```python
from build123d import *

# Parameters (mm, degrees)
F1_DEPTH    = 130
F2_T1_DEPTH = 154.4948974279
F3_T1_DEPTH = 154.4948974279
F4_R        = 5


# Not quite as in the source:
# - a fillet or chamfer that OpenCascade refuses, or shapes differently, is made with other operations: its cross-section is extruded or revolved along the edge and cut away or added


with BuildPart() as f1:
    # F0 (on Right) → F1 (new body)
    with BuildSketch(Plane.YZ):
        Polygon((1.0352761804, 3.8637033052), (0, 0), (120, 0), (120, 4), (5.2129014914, 4), (30.6586225483, 98.9647238196), (26.7949192431, 100), align=None)
        Polygon((-10, 0), (0, 0), (1.0352761804, 3.8637033052), (-10, 6.820596646), (-10, 4.0079755444), align=None)
    extrude(amount=F1_DEPTH)

    # F2: fillet of radius 5 on 1 edges, made by hand

    # F2_s2 → F2_t1 (cut)
    with BuildSketch(Plane.YZ.offset(-12.2474487139)):
        with BuildLine():
            ThreePointArc((30.6586225483, 98.9647238196), (27.4340422276, 98.0307814801), (25.5269700507, 95.2679491924))
            Line((25.5269700507, 95.2679491924), (26.7949192431, 100))
            Line((26.7949192431, 100), (30.6586225483, 98.9647238196))
        make_face()
    extrude(amount=F2_T1_DEPTH, mode=Mode.SUBTRACT)

    # F3: fillet of radius 5 on 1 edges, made by hand

    # F3_s2 → F3_t1 (cut)
    with BuildSketch(Plane.YZ.offset(-12.2474487139)):
        with BuildLine():
            ThreePointArc((115.1010205144, 4), (118.2632981746, 2.8729833462), (120, 0))
            Line((120, 0), (120, 4))
            Line((120, 4), (115.1010205144, 4))
        make_face()
    extrude(amount=F3_T1_DEPTH, mode=Mode.SUBTRACT)

    # F4
    f4_edges = [f1.edges().sort_by_distance(p)[0] for p in [
        (65, -10, 6.820597),
    ]]
    fillet(f4_edges, radius=F4_R)


solid = f1.part
```
Model file for the job. Use its own axes, mm. A direction names the side the tool comes from. Give positions to 0.01 mm unless a question says otherwise; leave off trailing zeros. Loops run counter-clockwise (first coordinate to the right, second up) from the corner with the lowest first, then second, coordinate; pieces in that order, holes last. Notation, with made-up numbers: (14, 14) -> (36, 14) arc R14 ccw to (36, 32) -> close; hole circle Ø1 at (-28.5, -13.5). An arc over 180 degrees is marked (long way). Use CSV: the item, a comma, the result in double quotes. Start each with the question number.
1) Slice it at A-A on x = 74. Give the cut face in (y, z).
2) Slice it at D-D on z = 22. Give the cut face in (x, y).
3) Tool access for faces 4 (the flat face through (0, 35, 2)), 5 (the flat face through (64.09, -1.3, 4.49)), 6 (the flat face through (64.09, 17.76, 50.82)): list every direction of +Z, -Z, +X, -X, +Y, -Y with a clear straight run to the whole face (end or side of a thin tool).
4) Flat gauge pins, fed straight in: pin 1 Ø3 at (x, y) = (36, 96.5) entering from +Z; pin 2 Ø4 at (x, z) = (97.5, 20.5) entering from +Y; pin 3 Ø3 at (x, z) = (70, 53) entering from -Y. Where does each tip first touch, or does it go through?
5) Mould opens along Z. For faces 1 (the flat face through (64, 61, 4)), 2 (the flat face through (64, 54, 0)), 3 (the cylindrical face through (64.09, 118.23, 2.9)) say: released by +Z, released by -Z, zero draft, split by the parting line, or undercut.
6) Slice it at B-B on y = 7. Give the cut face in (x, z), plus the area to 3 significant figures.
7) Slice it at C-C on y = 56. Give the cut face in (x, z).
8) Wall check: line 1 (Z direction, x = 86.5, y = 86); line 2 (Y direction, x = 78, z = 47); line 3 (Y direction, x = 63, z = 94). Give the ranges that are in metal, low to high.
Computed values:
1,outline,"(-10, 0) -> (120, 0) arc R5 ccw to (115.1, 4) -> (5.21, 4) -> (30.66, 98.96) arc R5 ccw to (25.53, 95.27) -> (1.04, 3.86) -> (-3.71, 5.13) arc R5 ccw to (-10, 0.3) -> close"
2,outline,"(0, 5.89) -> (130, 5.89) -> (130, 10.04) -> (0, 10.04) -> close"
3,face 4,"+Z, -Z, -X, +Y, -Y"
3,face 5,"+Z, +X, -X"
3,face 6,"+X, -X, +Y"
4,pin 1,"stops at z = 4"
4,pin 2,"stops at y = 10.17"
4,pin 3,"stops at y = 13.8"
5,face 1,"undercut"
5,face 2,"released by -Z"
5,face 3,"released by +Z"
6,outline,"(0, 0) -> (130, 0) -> (130, 4) -> (0, 4) -> close; (0, 10.67) -> (130, 10.67) -> (130, 26.12) -> (0, 26.12) -> close"
6,area,"2,530 mm^2"
7,outline,"(0, 0) -> (130, 0) -> (130, 4) -> (0, 4) -> close"
8,line 1,"z = 0 to 4"
8,line 2,"y = 12.59 to 16.73"
8,line 3,"y = 25.19 to 29.33"
